Geometry check sheet. Reference: the model listing, model coordinates, mm. Face numbers are marked on the shaded views. A direction names the side the tool comes from. Round coordinates to 2 decimals unless told otherwise and drop trailing zeros. Order: outer loops, then holes, each group sorted by start corner. A loop starts at its lowest first (then second) coordinate and runs counter-clockwise, first axis right, second up. Notation, with made-up numbers: (62.25, 44.25) -> (102.25, 44.25) arc R10 ccw to (102.25, 62.25) -> close; hole circle Ø5 at (-38.75, 64). An arc over 180 degrees is marked (long way). Use a Markdown table: item, result. Add a question column.
Item 1: Gauge pin test, flat ends, axial feed: pin 1 Ø3.5 at (x, y) = (-28, -24) entering from -Z; pin 2 Ø5 at (y, z) = (-14.5, 12.5) entering from -X; pin 3 Ø4.5 at (x, y) = (-15.5, -15.5) entering from +Z; pin 4 Ø1.6 at (x, z) = (-7, 1) entering from -Y. Record the tip position at first contact, or that the pin passes through.
Item 2: Sectioned sample at D-D, the plane y = -2. Record the cut outline in (x, z), and give its area (3 significant figures).
Item 3: Material ranges on probe 1 along Y at (x, z) = (-15.5, 0.6); probe 2 along Z at (x, y) = (-35, -24); probe 3 along Y at (x, z) = (0, 0.55), recorded low to high. Write a range as [from, to].
Item 4: Sectioned sample at A-A, the plane x = -35.5. Record the cut outline in (y, z), and give its area (3 significant figures).
Item 5: Sectioned sample at C-C, the plane x = 0. Record the cut outline in (y, z).
Item 6: Set-up check for the marked faces 4 and 5: record each of +Z, -Z, +X, -X, +Y, -Y from which the full face is reachable in a straight line by a thin tool's end or side.
Item 7: Mould release check, pull along Z, two halves, no side actions. Record for the marked faces 1, 2 and 3: pulls with the +Z half, pulls with the -Z half, needs draft (parallel to the pull), parting line crosses it, or undercut.
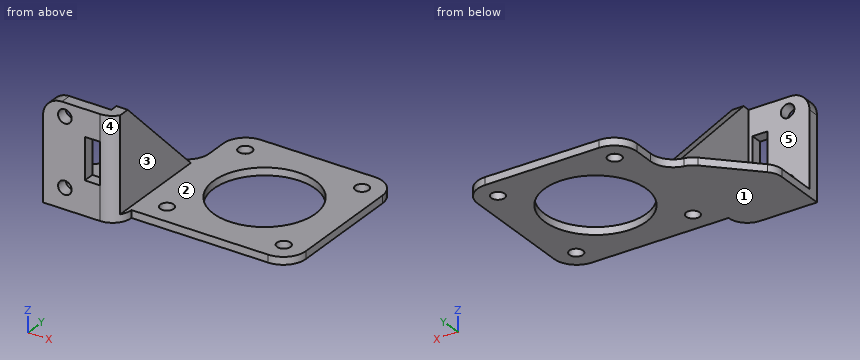
from build123d import *

# Parameters (mm, degrees)
F0_R         = 1.8
F0_R_2       = 13.5
F0_W         = 20.1372796029
F0_H         = 5
F1_DEPTH     = 2
F2_W         = 3
F2_H         = 30
F3_DEPTH     = 27
F4_W         = 16.1372796029
F4_H         = 3
F5_DEPTH     = 25
F6_R         = 1.8
F6_W         = 4
F6_H         = 11
F7_DEPTH     = 25
F8_SIZE      = 25
F9_SIZE      = 14
F10_R        = 4.99999
F11_T1_DEPTH = 2
F11_T3_DEPTH = 32


# Not quite as in the source:
# - a fillet or chamfer that OpenCascade refuses, or shapes differently, is made with other operations: its cross-section is extruded or revolved along the edge and cut away or added
# - a fillet or chamfer is up to 0.001 mm smaller than in the source, because OpenCascade refuses the exact size
# - a feature names something its author has since deleted; it is built from what else it names


with BuildPart() as f1:
    # F0 (on Top) → F1 (new body)
    with BuildSketch(Plane.XY):
        Polygon((21.15, -21.15), (21.15, 21.15), (-21.15, 21.15), (-21.15, 3.85), (-21.15, -21.15), align=None)
        with Locations((-15.5, -15.5)):
            Circle(F0_R, mode=Mode.SUBTRACT)
        with Locations((15.5, -15.5)):
            Circle(F0_R, mode=Mode.SUBTRACT)
        with Locations((-15.5, 15.5)):
            Circle(F0_R, mode=Mode.SUBTRACT)
        Circle(F0_R_2, mode=Mode.SUBTRACT)
        with Locations((15.5, 15.5)):
            Circle(F0_R, mode=Mode.SUBTRACT)
        Polygon((-21.15, -21.15), (-21.15, 3.85), (-41.3, 3.85), (-41.3, -21.15), (-21.1627203971, -21.15), align=None)
        with Locations((-31.2313601986, -23.65)):
            Rectangle(F0_W, F0_H)
    extrude(amount=F1_DEPTH)

    # F2 (on Top) → F3 (join)
    with BuildSketch(Plane.XY):
        with Locations((-23.6627203971, -11.15)):
            Rectangle(F2_W, F2_H)
    extrude(amount=F3_DEPTH)

    # F4 (on face) → F5 (join)
    with BuildSketch(Plane.XY.offset(2)):
        with Locations((-33.2313601986, -24.65)):
            Rectangle(F4_W, F4_H)
    extrude(amount=F5_DEPTH)

    # F6 (on face) → F7 (cut)
    with BuildSketch(Plane(origin=(0, -23.15, 0), x_dir=(-1, 0, 0), z_dir=(0, 1, 0))):
        with Locations((35.5, 5.5)):
            Circle(F6_R)
        with Locations((35.5, 23.5)):
            Circle(F6_R)
        with Locations((28.2, 14.5)):
            Rectangle(F6_W, F6_H)
    extrude(amount=-F7_DEPTH, mode=Mode.SUBTRACT)

    # F8
    f8_edges = [f1.edges().sort_by_distance(p)[0] for p in [
        (-23.66272, 3.85, 27),
    ]]
    chamfer(f8_edges, length=F8_SIZE)

    # F9
    f9_edges = [f1.edges().sort_by_distance(p)[0] for p in [
        (-41.3, 3.85, 1),
    ]]
    chamfer(f9_edges, length=F9_SIZE)

    # F10 (radius 5 in the source; OpenCascade refuses exactly that, so slightly less here)
    f10_edges = [f1.edges().sort_by_distance(p)[0] for p in [
        (-41.3, -10.15, 1),
        (-27.3, 3.85, 1),
        (-21.16272, -26.15, 1),
        (-41.3, -24.65, 27),
    ]]
    fillet(f10_edges, radius=F10_R)

    # F11: fillet of radius 6 on 4 edges, made by hand

    # F11_s2 → F11_t1 (join)
    with BuildSketch(Plane.XY):
        with BuildLine():
            ThreePointArc((-26.1021461366, 3.7731598692), (-22.5517871308, 5.8265464621), (-21.15, 9.6809515277))
            Line((-21.15, 9.6809515277), (-20.55, 9.6809515277))
            Line((-20.55, 9.6809515277), (-20.55, 3.85))
            Line((-20.55, 3.85), (-21.15, 3.25))
            ThreePointArc((-21.15, 3.25), (-25.2289363303, 3.25), (-25.9973607503, 3.1823807033))
            Line((-25.9973607503, 3.1823807033), (-26.1021461366, 3.7731598692))
        make_face()
    extrude(amount=F11_T1_DEPTH)

    # F11_s4 → F11_t3 (cut)
    with BuildSketch(Plane.XY.offset(-15)):
        with BuildLine():
            ThreePointArc((21.15, -15.15), (19.3926406871, -19.3926406871), (15.15, -21.15))
            Line((15.15, -21.15), (21.15, -21.15))
            Line((21.15, -21.15), (21.15, -15.15))
        make_face()
        with BuildLine():
            ThreePointArc((15.15, 21.15), (19.3926406871, 19.3926406871), (21.15, 15.15))
            Line((21.15, 15.15), (21.15, 21.15))
            Line((21.15, 21.15), (15.15, 21.15))
        make_face()
        with BuildLine():
            ThreePointArc((-21.15, 15.15), (-19.3926406871, 19.3926406871), (-15.15, 21.15))
            Line((-15.15, 21.15), (-21.15, 21.15))
            Line((-21.15, 21.15), (-21.15, 15.15))
        make_face()
    extrude(amount=F11_T3_DEPTH, mode=Mode.SUBTRACT)


solid = f1.part
Found:
| question | item | result |
|---|---|---|
| 1 | pin 1 | stops at z = 0 |
| 1 | pin 2 | stops at x = -25.16 |
| 1 | pin 3 | stops at z = 2 |
| 1 | pin 4 | stops at y = -21.15 |
| 2 | outline | (-33.15, 0) -> (-13.35, 0) -> (-13.35, 2) -> (-22.16, 2) -> (-22.16, 7.85) -> (-25.16, 7.85) -> (-25.16, 2) -> (-33.15, 2) -> close; (13.35, 0) -> (21.15, 0) -> (21.15, 2) -> (13.35, 2) -> close |
| 2 | area | 72.7 mm2 |
| 3 | probe 1 | y = [-21.15, -17.3], [-13.7, 13.7], [17.3, 21.14] |
| 3 | probe 2 | z = [0, 3.77], [7.23, 21.77], [25.23, 27] |
| 3 | probe 3 | y = [-21.15, -13.5], [13.5, 21.15] |
| 4 | outline | (-26.15, 0) -> (-4.35, 0) -> (-4.35, 2) -> (-23.15, 2) -> (-23.15, 3.7) -> (-26.15, 3.7) -> close; (-26.15, 7.3) -> (-23.15, 7.3) -> (-23.15, 21.7) -> (-26.15, 21.7) -> close; (-26.15, 25.3) -> (-23.15, 25.3) -> (-23.15, 27) -> (-26.15, 27) -> close |
| 4 | area | 97.0 mm2 |
| 5 | outline | (-21.15, 0) -> (-13.5, 0) -> (-13.5, 2) -> (-21.15, 2) -> close; (13.5, 0) -> (21.15, 0) -> (21.15, 2) -> (13.5, 2) -> close |
| 6 | face 4 | +Z, -Z, +X, -Y |
| 6 | face 5 | +Z, -X, +Y |
| 7 | face 1 | pulls with the -Z half |
| 7 | face 2 | pulls with the +Z half |
| 7 | face 3 | needs draft |
